```python
from build123d import *

# Parameters (mm, degrees)
F1_DEPTH = 60
F2_R     = 5
F3_SIZE  = 5
F4_SIZE  = 5
F5_R     = 28.204224
F6_DEPTH = 30


with BuildPart() as f1:
    # F0 (on Front) → F1 (new body)
    with BuildSketch(Plane.XZ):
        with BuildLine():
            Line((31.411576, 50.537112), (-28.546256, 50.537112))
            ThreePointArc((-28.546256, 50.537112), (-42.32879, 44.828199), (-48.037703, 31.045665))
            Line((-48.037703, 31.045665), (-48.037703, -49.462888))
            Line((-48.037703, -49.462888), (31.524516, -49.462888))
            ThreePointArc((31.524516, -49.462888), (45.97621, -43.476801), (51.962297, -29.025107))
            Line((51.962297, -29.025107), (51.962297, 29.986391))
            Line((51.962297, 29.986391), (51.962297, 50.537112))
            Line((51.962297, 50.537112), (31.411576, 50.537112))
        make_face()
    extrude(amount=F1_DEPTH)

    # F2
    f2_edges = [f1.edges().sort_by_distance(p)[0] for p in [
        (-42.32879, 0, 44.828199),
        (-48.037703, 0, -9.208612),
        (-8.256593, 0, -49.462888),
        (45.97621, 0, -43.476801),
        (51.962297, 0, 10.756002),
        (11.708021, 0, 50.537112),
    ]]
    fillet(f2_edges, radius=F2_R)

    # F3
    f3_edges = [f1.edges().sort_by_distance(p)[0] for p in [
        (11.708021, -60, 50.537112),
        (-42.32879, -60, 44.828199),
        (-48.037703, -60, -9.208612),
        (-8.256593, -60, -49.462888),
        (45.97621, -60, -43.476801),
        (51.962297, -60, 10.756002),
    ]]
    chamfer(f3_edges, length=F3_SIZE)

    # F4
    f4_edges = [f1.edges().sort_by_distance(p)[0] for p in [
        (-43.037703, -60, -6.708612),
        (-5.756593, -60, -44.462888),
        (-38.793256, -60, 41.292665),
        (42.440676, -60, -39.941267),
        (9.208021, -60, 45.537112),
        (46.962297, -60, 8.256002),
    ]]
    chamfer(f4_edges, length=F4_SIZE)

    # F5 (on face) → F6 (join)
    with BuildSketch(Plane.XZ.offset(60)):
        Circle(F5_R)
    extrude(amount=F6_DEPTH)


solid = f1.part
```
The model under review builds one solid part; all positions refer to its coordinate system, in mm. A direction names the side the tool comes from. Give positions to 0.01 mm unless a question says otherwise; leave off trailing zeros. Loops run counter-clockwise (first coordinate to the right, second up) from the corner with the lowest first, then second, coordinate; pieces in that order, holes last. Notation, with made-up numbers: (55.5, 49) - (66.5, 49) arc R16 cw to (66.5, 63) - close; hole circle Ø2 at (35.25, -36). An arc over 180 degrees is marked (long way). Answer as a JSON object with one key per item and string values.
Q1. Add section C-C on y = -26. State the section outline as (x, z) points, plus the area to 3 significant figures.
Worked out:
{"outline": "(-48.04, -49.46) - (31.52, -49.46) arc R20.44 ccw to (51.96, -29.03) - (51.96, 50.54) - (-28.55, 50.54) arc R19.49 ccw to (-48.04, 31.05) - close", "area": "9,830 mm^2"}
Q2. For faces 1 (the flat face through (10, -60, 28)), 2 (the flat face through (-8.071, -58.207, -43.79)), list the 3-axis set-ups (+Z, -Z, +X, -X, +Y, -Y) from which the entire face can be reached by the end or side of a thin tool; tool diameter is ignored.
Worked out:
{"face 1": "-Y", "face 2": "-Z, +X, -X, -Y"}
Q3. Add section B-B on x = 0. State the section outline as (y, z) points, plus the area to 3 significant figures.
Worked out:
{"outline": "(-90, -28.2) - (-60, -28.2) - (-60, -39.46) - (-56.46, -48) - (-55, -49.46) - (-5, -49.46) arc R5 ccw to (0, -44.46) - (0, 45.54) arc R5 ccw to (-5, 50.54) - (-55, 50.54) - (-56.46, 49.07) - (-60, 40.54) - (-60, 28.2) - (-90, 28.2) - close", "area": "7,640 mm^2"}
Q4. Insertion check: pin 1 (8 mm diameter, centred on x = -27, y = -59.5, fed in from +Z); pin 2 (5 mm diameter, centred on y = -62, z = -20.5, fed in from +X); pin 3 (1.5 mm diameter, centred on x = 34.5, y = -50.5, fed in from -Z). Each pin has a flat end and moves straight along its axis. Give the tip position at first contact, or say it passes through.
Worked out:
{"pin 1": "stops at z = 50.04", "pin 2": "stops at x = 43.17", "pin 3": "stops at z = -49.34"}
Q5. Add section A-A on z = 0. State the section outline as (x, y) points, plus the area to 3 significant figures.
Worked out:
{"outline": "(-48.04, -55) - (-46.57, -56.46) - (-38.04, -60) - (-28.2, -60) - (-28.2, -90) - (28.2, -90) - (28.2, -60) - (41.96, -60) - (50.5, -56.46) - (51.96, -55) - (51.96, -5) arc R5 ccw to (46.96, 0) - (-43.04, 0) arc R5 ccw to (-48.04, -5) - close", "area": "7,640 mm^2"}
Q6. To check wall thickness, follow line 1 along Y through (x, z) = (21, 29); line 2 along Z through (x, y) = (-32, -17); line 3 along Z through (x, y) = (-3.5, -57.5). State the ranges of each line that lie inside material, in increasing order.
Worked out:
{"line 1": "y = -60 to 0", "line 2": "z = -49.46 to 50.23", "line 3": "z = -45.5 to 46.57"}
